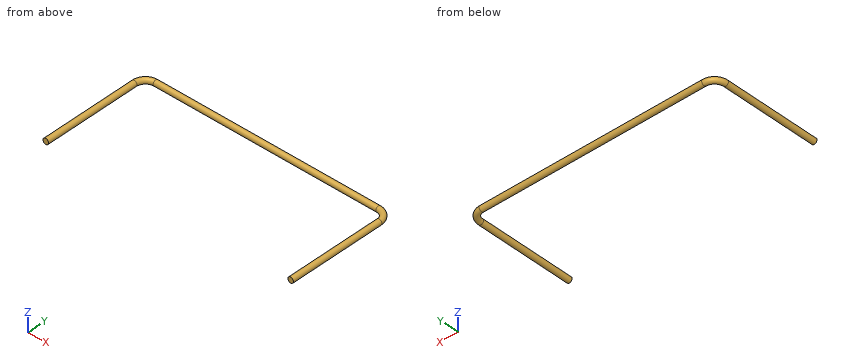
from build123d import *

# Parameters (mm, degrees)
ESQUISSE2_R = 0.5


with BuildPart() as part:
    # Balayage1: sweep along a path in Esquisse1
    with BuildLine(Plane.XY) as balayage1_path:
        Line((-8.67886357, 0), (-8.67886357, 17.12919258))
        ThreePointArc((-8.67886357, 17.12919258), (-8.093077132, 18.543406142), (-6.67886357, 19.12919258))
        Line((-6.67886357, 19.12919258), (33.32113643, 19.12919258))
        ThreePointArc((33.32113643, 19.12919258), (34.735349992, 18.543406142), (35.32113643, 17.12919258))
        Line((35.32113643, 17.12919258), (35.32113643, 0))
    # Esquisse2 → Balayage1 (sweep)
    with BuildSketch(Plane(origin=(0, 0, 0), x_dir=(1, 0, 0), z_dir=(0, 1, 0))):
        with Locations((-8.67886357, 0)):
            Circle(ESQUISSE2_R)
    sweep(path=balayage1_path.line)


solid = part.part
Geometry check sheet. Reference: the model listing, model coordinates, mm. Round coordinates to 2 decimals unless told otherwise and drop trailing zeros. Loops run counter-clockwise (first coordinate to the right, second up) from the corner with the lowest first, then second, coordinate; pieces in that order, holes last.
Item 1: Thickness scan on line 1 (X direction, y = 3.5, z = -0.1); line 2 (Y direction, x = 7, z = 0); line 3 (X direction, y = 8.5, z = -0.2). Record the ranges inside material, lowest first.
Item 2: Cross-section at A-A on z = 0. Record the boundary of the cut face in (x, y), then the cut area to 3 significant figures.
Item 3: Gauge pin test, flat end, axial feed: pin 1 (6 mm diameter, centred on x = 18.5, y = 13, fed in from +Z). Record the tip position at first contact, or that the pin passes through.
Item 4: Cross-section at B-B on y = 7.25. Record the boundary of the cut face in (x, z).
Item 5: Cross-section at C-C on x = 8.5. Record the boundary of the cut face in (y, z), then the cut area to 3 significant figures.
Answer sheet:
1. line 1: x = -9.17 to -8.19, 34.83 to 35.81
1. line 2: y = 18.63 to 19.63
1. line 3: x = -9.14 to -8.22, 34.86 to 35.78
2. outline: (-9.18, 0) - (-8.18, 0) - (-8.18, 17.13) arc R1.5 cw to (-6.68, 18.63) - (33.32, 18.63) arc R1.5 cw to (34.82, 17.13) - (34.82, 0) - (35.82, 0) - (35.82, 17.13) arc R2.5 ccw to (33.32, 19.63) - (-6.68, 19.63) arc R2.5 ccw to (-9.18, 17.13) - close
2. area: 80.5 mm2
3. pin 1: passes through
4. outline: circle Ø1 at (-8.68, 0); circle Ø1 at (35.32, 0)
5. outline: circle Ø1 at (19.13, 0)
5. area: 0.785 mm2
